Answer from the drawing. Dimensions are ordinates in mm from the lowest x, y and z of the part. A direction names the side the tool comes from. Round coordinates to 2 decimals unless told otherwise and drop trailing zeros. Write each loop counter-clockwise with the first axis right and the second up, starting at its lowest first coordinate (ties: lowest second). Pieces come first, ordered by that corner, then holes. Notation, with made-up numbers: (32.25, -32.5) -> (52.25, -32.5) arc R22 ccw to (52.25, -20.5) -> close; hole circle Ø3 at (19.25, 5.25). An arc over 180 degrees is marked (long way). Return JSON: item names as keys, results as strings. Group by question number.
(1) A cutting plane is placed at B-B on z = 3. Give the vertices of the cut face in (x, y).
(2) A cutting plane is placed at D-D on z = 6.25. Give the vertices of the cut face in (x, y).
(3) Given pin 1 (3 mm diameter, centred on x = 5.5, y = 4, fed in from +Z); pin 2 (5 mm diameter, centred on x = 2.5, z = 7.5, fed in from -Y); pin 3 (2.5 mm diameter, centred on x = 4, y = 3.5, fed in from -Z); pin 4 (1.3 mm diameter, centred on y = 4.5, z = 4, fed in from -X), each flat-ended and moving along its own axis, determine where each tip first touches the part or whether it passes through.
(4) The mould has two halves that part along X. Classify the marked faces 1, 2, 3 and 4: released by +X, released by -X, zero draft, split by the parting line, or undercut.
(5) Straight lines are drawn through the part: line 1 (Y direction, x = 6.5, z = 6.75); line 2 (X direction, y = 1.25, z = 5.75) (1 decimal); line 3 (Z direction, x = 5, y = 4.25) (1 decimal). For each, find the intervals that lie inside material, in ascending order.
(6) A cutting plane is placed at C-C on y = 5.25. Give the vertices of the cut face in (x, z).
(7) For the marked faces 5, 6 and 7, determine the directions among +Z, -Z, +X, -X, +Y, -Y from which every point of the face is accessible in a straight line to the end or side of a thin tool.
(8) A cutting plane is placed at A-A on x = 3. Give the vertices of the cut face in (y, z).
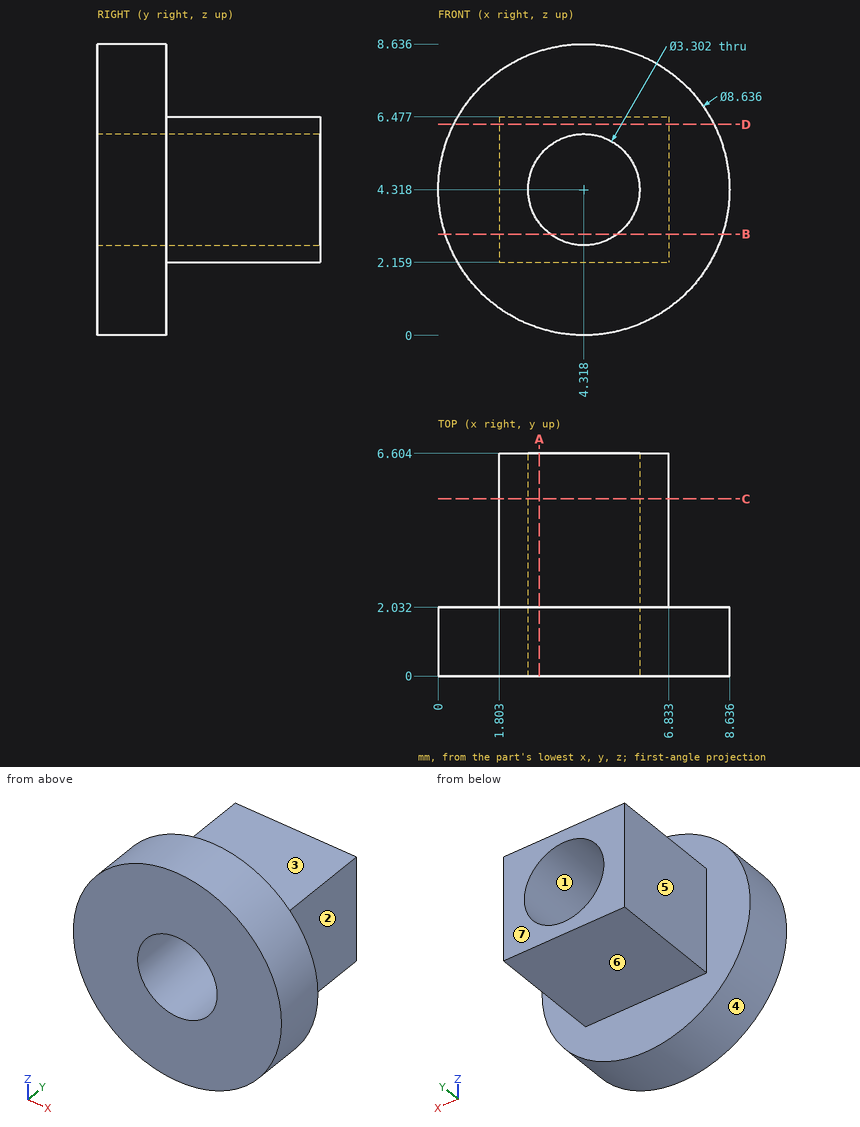
Checks:
{
 "1": {"outline": "(0.21, 0) -> (3.32, 0) -> (3.32, 6.6) -> (1.8, 6.6) -> (1.8, 2.03) -> (0.21, 2.03) -> close; (5.31, 0) -> (8.43, 0) -> (8.43, 2.03) -> (6.83, 2.03) -> (6.83, 6.6) -> (5.31, 6.6) -> close"},
 "2": {"outline": "(0.46, 0) -> (8.18, 0) -> (8.18, 2.03) -> (6.83, 2.03) -> (6.83, 6.6) -> (1.8, 6.6) -> (1.8, 2.03) -> (0.46, 2.03) -> close"},
 "3": {"pin 1": "stops at z = 6.48", "pin 2": "stops at y = 0", "pin 3": "stops at z = 2.16", "pin 4": "stops at x = 1.8"},
 "4": {"face 1": "undercut", "face 2": "released by +X", "face 3": "zero draft", "face 4": "split by the parting line"},
 "5": {"line 1": "y = 0 to 2.03", "line 2": "x = 0.2 to 3.5, 5.1 to 8.4", "line 3": "z = 2.2 to 2.8, 5.8 to 6.5"},
 "6": {"outline": "(1.8, 2.16) -> (6.83, 2.16) -> (6.83, 6.48) -> (1.8, 6.48) -> close; hole circle Ø3.3 at (4.32, 4.32)"},
 "7": {"face 5": "+Z, -Z, -X, +Y", "face 6": "-Z, +X, -X, +Y", "face 7": "+Z, -Z, +X, -X, +Y"},
 "8": {"outline": "(0, 0.21) -> (2.03, 0.21) -> (2.03, 2.16) -> (6.6, 2.16) -> (6.6, 3.32) -> (0, 3.32) -> close; (0, 5.31) -> (6.6, 5.31) -> (6.6, 6.48) -> (2.03, 6.48) -> (2.03, 8.43) -> (0, 8.43) -> close"}
}
